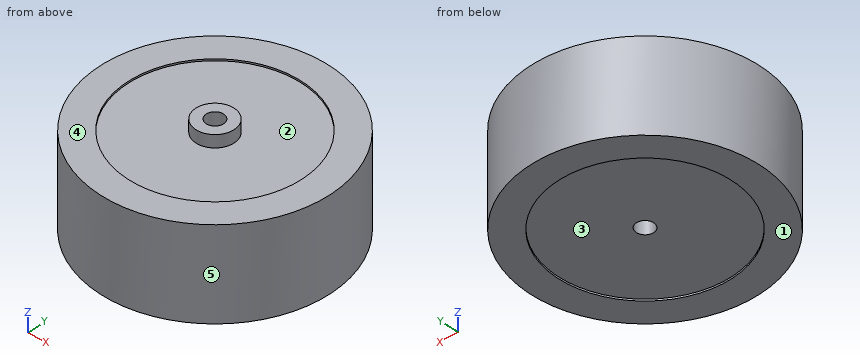
```python
from build123d import *

# Parameters (mm, degrees)
SCHIZZO1_R                        = 33
SCHIZZO1_R_2                      = 25
ESTRUSIONE_ESTRUSIONE1_DEPTH      = 13
ESTRUSIONE_ESTRUSIONE1_DEPTH_BACK = 13
SCHIZZO1_3_R                      = 25
SCHIZZO1_3_R_2                    = 2.5
ESTRUSIONE_ESTRUSIONE2_DEPTH      = 12.5
ESTRUSIONE_ESTRUSIONE2_DEPTH_BACK = 12.5
SCHIZZO2_R                        = 5.5
SCHIZZO2_R_2                      = 2.5
ESTRUSIONE_ESTRUSIONE3_DEPTH      = 3.5


with BuildPart() as part:
    # Schizzo1 → Estrusione-Estrusione1 (new body, two sides)
    with BuildSketch(Plane.XY) as estrusione_estrusione1_sk:
        Circle(SCHIZZO1_R)
        Circle(SCHIZZO1_R_2, mode=Mode.SUBTRACT)
    extrude(amount=ESTRUSIONE_ESTRUSIONE1_DEPTH)
    extrude(estrusione_estrusione1_sk.sketch, amount=-ESTRUSIONE_ESTRUSIONE1_DEPTH_BACK)

    # Schizzo1_3 → Estrusione-Estrusione2 (add, two sides)
    with BuildSketch(Plane.XY) as estrusione_estrusione2_sk:
        Circle(SCHIZZO1_3_R)
        Circle(SCHIZZO1_3_R_2, mode=Mode.SUBTRACT)
    extrude(amount=ESTRUSIONE_ESTRUSIONE2_DEPTH)
    extrude(estrusione_estrusione2_sk.sketch, amount=-ESTRUSIONE_ESTRUSIONE2_DEPTH_BACK)

    # Schizzo2 → Estrusione-Estrusione3 (add)
    with BuildSketch(Plane.XY.offset(12.5)):
        Circle(SCHIZZO2_R)
        Circle(SCHIZZO2_R_2, mode=Mode.SUBTRACT)
    extrude(amount=ESTRUSIONE_ESTRUSIONE3_DEPTH)


solid = part.part
```
Verification items for the finished model (mm, model axes). Face numbers are marked on the shaded views. A direction names the side the tool comes from. Coordinates: 2 decimals unless noted, no trailing zeros. Write each loop counter-clockwise with the first axis right and the second up, starting at its lowest first coordinate (ties: lowest second). Pieces come first, ordered by that corner, then holes. Notation, with made-up numbers: M -39.75,40.5 L -1.75,40.5 A24 cw -1.75,56.5 Z; hole C 85.5,11.5 d6. An arc over 180 degrees is marked long. One line per item, written item: value.
Item 1: Scan lines: line 1 along Y through (x, z) = (0, -12.6); line 2 along Z through (x, y) = (-25.5, 8.5); line 3 along Y through (x, z) = (0, -3.5). Record each from-to range of solid material in increasing order.
Check sheet entries:
line 1: y = -33 to -25, 25 to 33
line 2: z = -13 to 13
line 3: y = -33 to -2.5, 2.5 to 33
Item 2: Section check C-C, the plane z = 3.25. Record the boundary of the cut face in (x, y), plus the area to 3 significant figures.
Check sheet entries:
outline: C 0,0 d66; hole C 0,0 d5
area: 3,400 mm^2
Item 3: Mould release check, pull along X, two halves, no side actions. Record for the marked faces 3, 4 and 5: pulls with the +X half, pulls with the -X half, needs draft (parallel to the pull), parting line crosses it, or undercut.
Check sheet entries:
face 3: undercut
face 4: needs draft
face 5: parting line crosses it
Item 4: Section check D-D, the plane x = -11. Record the boundary of the cut face in (y, z).
Check sheet entries:
outline: M -31.11,-13 L -22.45,-13 L -22.45,-12.5 L 22.45,-12.5 L 22.45,-13 L 31.11,-13 L 31.11,13 L 22.45,13 L 22.45,12.5 L -22.45,12.5 L -22.45,13 L -31.11,13 Z
Item 5: Section check A-A, the plane x = 0. Record the boundary of the cut face in (y, z), plus the area to 3 significant figures.
Check sheet entries:
outline: M -33,-13 L -25,-13 L -25,-12.5 L -2.5,-12.5 L -2.5,16 L -5.5,16 L -5.5,12.5 L -25,12.5 L -25,13 L -33,13 Z; M 2.5,-12.5 L 25,-12.5 L 25,-13 L 33,-13 L 33,13 L 25,13 L 25,12.5 L 5.5,12.5 L 5.5,16 L 2.5,16 Z
area: 1,560 mm^2
Item 6: Gauge pin test, flat ends, axial feed: pin 1 Ø4 at (y, z) = (-24.5, 2) entering from +X; pin 2 Ø2 at (x, y) = (-1.5, -11) entering from +Z; pin 3 Ø6 at (y, z) = (-25.5, 7) entering from -X; pin 4 Ø8 at (y, z) = (1.5, -3) entering from -X. Record the tip position at first contact, or that the pin passes through.
Check sheet entries:
pin 1: stops at x = 24.14
pin 2: stops at z = 12.5
pin 3: stops at x = -24.14
pin 4: stops at x = -33
Item 7: Access from +Z, -Z, +X, -X, +Y, -Y to the whole of each face (thin tool, end or side, straight path). Record for the marked faces 1 and 2.
Check sheet entries:
face 1: -Z, +X, -X, +Y, -Y
face 2: +Z
